from build123d import *

# Parameters (mm, degrees)
SKETCH_1_R          = 9.5
SKETCH_1_R_2        = 2
EXTRUDE_1_DEPTH     = 6
SKETCH_2_W          = 12
SKETCH_2_H          = 24
SKETCH_2_W_2        = 10
SKETCH_2_H_2        = 10
CUT_EXTRUDE_1_DEPTH = 6
FILLET_1_R          = 3
SKETCH_3_R          = 9.5
SKETCH_3_R_2        = 8
EXTRUDE_3_DEPTH     = 1


with BuildPart() as part:
    # 草图1 → 凸台-拉伸1 (new body)
    with BuildSketch(Plane.XY):
        with BuildLine():
            Line((-15, -64), (-15, 64))
            ThreePointArc((-15, 64), (0, 79), (15, 64))
            Line((15, 64), (15, -64))
            ThreePointArc((15, -64), (0, -79), (-15, -64))
        make_face()
        with Locations((0, 64)):
            Circle(SKETCH_1_R, mode=Mode.SUBTRACT)
        with Locations((0, -54)):
            Circle(SKETCH_1_R_2, mode=Mode.SUBTRACT)
        with Locations((10, -64)):
            Circle(SKETCH_1_R_2, mode=Mode.SUBTRACT)
        with Locations((0, -74)):
            Circle(SKETCH_1_R_2, mode=Mode.SUBTRACT)
        with Locations((-10, -64)):
            Circle(SKETCH_1_R_2, mode=Mode.SUBTRACT)
    extrude(amount=EXTRUDE_1_DEPTH)

    # 草图2 → 切除-拉伸1 (cut)
    with BuildSketch(Plane.XY.offset(6)):
        with Locations((0, 34)):
            Rectangle(SKETCH_2_W, SKETCH_2_H)
        Rectangle(SKETCH_2_W, SKETCH_2_H)
        with Locations((0, -34)):
            Rectangle(SKETCH_2_W, SKETCH_2_H)
        with Locations((0, -64)):
            Rectangle(SKETCH_2_W_2, SKETCH_2_H_2)
    extrude(amount=-CUT_EXTRUDE_1_DEPTH, mode=Mode.SUBTRACT)

    # 圆角1
    fillet_1_edges = [part.edges().sort_by_distance(p)[0] for p in [
        (5, -59, 3),
        (5, -69, 3),
        (-5, -69, 3),
        (-5, -59, 3),
    ]]
    fillet(fillet_1_edges, radius=FILLET_1_R)

    # 草图3 → 凸台-拉伸3 (add)
    with BuildSketch(Plane(origin=(0, 0, 0), x_dir=(-1, 0, 0), z_dir=(0, 0, -1))):
        with Locations((0, 64)):
            Circle(SKETCH_3_R)
        with Locations((0, 64)):
            Circle(SKETCH_3_R_2, mode=Mode.SUBTRACT)
    extrude(amount=-EXTRUDE_3_DEPTH)


solid = part.part
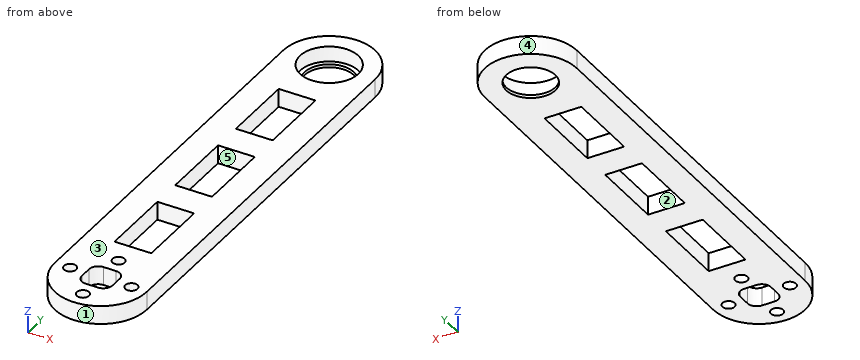
Geometry: final body of the model. Coordinates: model frame, mm. Face numbers are marked on the shaded views. A direction names the side the tool comes from. Give positions to 0.01 mm unless a question says otherwise; leave off trailing zeros. Loops run counter-clockwise (first coordinate to the right, second up) from the corner with the lowest first, then second, coordinate; pieces in that order, holes last. Notation, with made-up numbers: M 21,46.25 L 26,46.25 A38 ccw 26,85.25 Z; hole C 24.25,-10.75 d10. An arc over 180 degrees is marked long. Put each result on its own line as item: value. Start each with the question number.
1) Cut plane A-A (y = -54). Output: boundary loops of the cut face in (x, z), then the cut area to 3 significant figures.
2) Cut plane B-B (x = 0). Give the number of separate pieces and of enclosed holes in the cut face, then the cut area to 3 significant figures.
3) Access query for the marked faces 1 and 2. Directions: +Z, -Z, +X, -X, +Y, -Y. A direction counts if a zero-diameter tool reaches every point of the face in a straight line with its end or side. Return the directions, or none.
4) Cut plane D-D (y = 62.5). Output: boundary loops of the cut face in (x, z).
5) Ray query, line 1 along X through (y, z) = (-23.5, 4); line 2 along X through (y, z) = (57, 1.1); line 3 along X through (y, z) = (-69.5, 4.1). Return the intervals inside material, ascending.
6) Cut plane C-C (y = -35). Output: boundary loops of the cut face in (x, z), then the cut area to 3 significant figures.
7) Contact query for flat-ended pins moving along their axis: pin 1 (3 mm diameter, centred on x = 2, z = 2, fed in from -Y); pin 2 (3 mm diameter, centred on x = 0, y = -74, fed in from -Z) (3 decimals); pin 3 (1.2 mm diameter, centred on x = -0.5, z = 3, fed in from +Y); pin 4 (1 mm diameter, centred on x = -9.5, z = 3, fed in from +Y). Output: stop coordinate, or through.
8) Pull-direction query (X, two-part tool) for the marked faces 3, 4 and 5; classes: pulls with the +X half, pulls with the -X half, needs draft (parallel to the pull), parting line crosses it, or undercut.
Verdict:
1. outline: M -15,0 L -2,0 L -2,6 L -15,6 Z; M 2,0 L 15,0 L 15,6 L 2,6 Z
1. area: 156 mm2
2. separate pieces: 8
2. enclosed holes: 0
2. area: 297 mm2
3. face 1: +Z, -Z, -Y
3. face 2: +Z, -Z
4. outline: M -15,0 L -7.86,0 L -7.86,1 L -9.38,1 L -9.38,6 L -15,6 Z; M 7.86,0 L 15,0 L 15,6 L 9.38,6 L 9.38,1 L 7.86,1 Z
5. line 1: -15 to -6, 6 to 15
5. line 2: -15 to -6.42, 6.42 to 15
5. line 3: -13.96 to 13.96
6. outline: M -15,0 L -6,0 L -6,6 L -15,6 Z; M 6,0 L 15,0 L 15,6 L 6,6 Z
6. area: 108 mm2
7. pin 1: y = -78.99
7. pin 2: through
7. pin 3: y = 79
7. pin 4: y = 76
8. face 3: needs draft
8. face 4: parting line crosses it
8. face 5: undercut
